from build123d import *

# Parameters (mm, degrees)
F0_W     = 273.05
F0_H     = 114.3
F1_DEPTH = 19.05
F2_R     = 25.4
F3_DEPTH = 25.4
F4_W     = 127.1476745605
F4_H     = 61.7186785519
F5_DEPTH = 25.4
F7_DEPTH = 25.4


with BuildPart() as f1:
    # F0 (on Front) → F1 (new body)
    with BuildSketch(Plane.XZ):
        with Locations((136.525, 57.15)):
            Rectangle(F0_W, F0_H)
    extrude(amount=F1_DEPTH)

    # F2 (on face) → F3 (cut)
    with BuildSketch(Plane.XZ.offset(19.05)):
        with Locations((50.8, 50.8)):
            Circle(F2_R)
    extrude(amount=-F3_DEPTH, mode=Mode.SUBTRACT)

    # F4 (on face) → F5 (cut)
    with BuildSketch(Plane.XZ.offset(19.05)):
        with Locations((156.7656248808, 83.440660724)):
            Rectangle(F4_W, F4_H)
    extrude(amount=-F5_DEPTH, mode=Mode.SUBTRACT)

    # F6 (on face) → F7 (cut)
    with BuildSketch(Plane.XZ.offset(19.05)):
        Polygon((93.1917876005, 52.5813214481), (93.1917876005, 66.1489069462), (71.0378619315, 66.1489069462), (76.137460289, 52.5813214481), align=None)
    extrude(amount=-F7_DEPTH, mode=Mode.SUBTRACT)


solid = f1.part
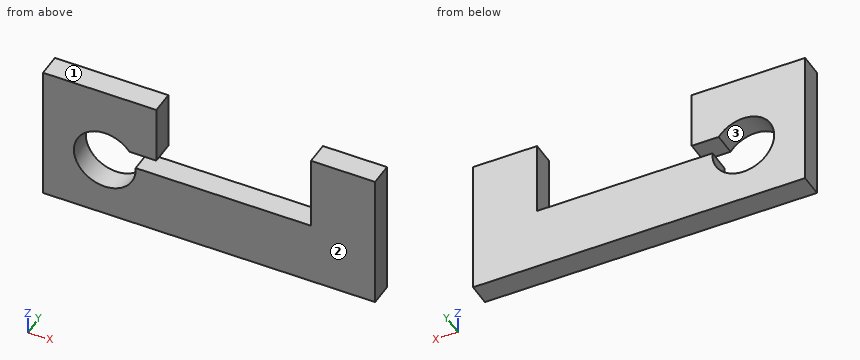
Part model, mm, in its own coordinate system. Face numbers are marked on the shaded views. Coordinates: 2 decimals unless noted, no trailing zeros. Order: outer loops, then holes, each group sorted by start corner. A loop starts at its lowest first (then second) coordinate and runs counter-clockwise, first axis right, second up. Notation, with made-up numbers: M 73,46.5 L 123,46.5 A24 ccw 123,82.5 Z; hole C 54,53.5 d5. An arc over 180 degrees is marked long. Use a Markdown table: item, result.
(1) Pull direction Z, two halves, no side cores. Call the marked faces 1, 2 and 3: released by +Z, released by -Z, zero draft, split by the parting line, or undercut.
A:
| item | result |
|---|---|
| face 1 | released by +Z |
| face 2 | zero draft |
| face 3 | undercut |
(2) Cut at D-D on x = 131.5. Write the cut outline in (y, z).
A:
| item | result |
|---|---|
| outline | M -19.05,0 L 0,0 L 0,52.58 L -19.05,52.58 Z |
(3) Cut at A-A on x = 50.8. Write the cut outline in (y, z).
A:
| item | result |
|---|---|
| outline | M -19.05,0 L 0,0 L 0,25.4 L -19.05,25.4 Z; M -19.05,76.2 L 0,76.2 L 0,114.3 L -19.05,114.3 Z |
(4) Flat gauge pin, fed straight in: pin 1 (4 mm diameter, centred on x = 131, y = -14.5, fed in from +Z). Where does the tip first touch, or does it go through?
A:
| item | result |
|---|---|
| pin 1 | stops at z = 52.58 |
(5) Cut at B-B on z = 50. Write the cut outline in (x, y).
A:
| item | result |
|---|---|
| outline | M 0,-19.05 L 25.41,-19.05 L 25.41,0 L 0,0 Z; M 76.19,-19.05 L 273.05,-19.05 L 273.05,0 L 76.19,0 Z |
(6) Probe L1, parallel to Z at x = 50.8, y = -7; L2, parallel to X at y = -6.5, z = 50.8; L3, parallel to X at y = -10.25, z = 106. List the from-to ranges inside material, lowest first.
A:
| item | result |
|---|---|
| L1 | z = 0 to 25.4, 76.2 to 114.3 |
| L2 | x = 0 to 25.4, 76.2 to 273.05 |
| L3 | x = 0 to 93.19, 220.34 to 273.05 |
(7) Cut at C-C on y = -11.25. Write the cut outline in (x, z).
A:
| item | result |
|---|---|
| outline | M 0,0 L 273.05,0 L 273.05,114.3 L 220.34,114.3 L 220.34,52.58 L 76.14,52.58 A25.4 cw long 71.04,66.15 L 93.19,66.15 L 93.19,114.3 L 0,114.3 Z |
